from build123d import *

# Parameters (mm, degrees)
SKETCH1_W           = 60
SKETCH1_H           = 40
BOSS_EXTRUDE1_DEPTH = 6
SKETCH3_R           = 1.15
CUT_EXTRUDE2_DEPTH  = 73.360210061
SKETCH12_W          = 25
SKETCH12_H          = 54
CUT_EXTRUDE10_DEPTH = 4
CUT_EXTRUDE11_DEPTH = 2.8
FILLET1_R           = 1
SKETCH15_W          = 9
SKETCH15_H          = 4
CUT_EXTRUDE13_DEPTH = 1.8
SKETCH16_W          = 4
SKETCH16_H          = 5
BOSS_EXTRUDE2_DEPTH = 7
SKETCH17_W          = 2
SKETCH17_H          = 2
SKETCH17_W_2        = 1.8
SKETCH17_H_2        = 7
BOSS_EXTRUDE3_DEPTH = 5


with BuildPart() as part:
    # Sketch1 → Boss-Extrude1 (new body)
    with BuildSketch(Plane(origin=(0, 0, 0), x_dir=(0, 1, 0), z_dir=(0, 0, 1))):
        with Locations((30, -20)):
            Rectangle(SKETCH1_W, SKETCH1_H)
    extrude(amount=BOSS_EXTRUDE1_DEPTH)

    # Sketch3 → Cut-Extrude2 (cut, through all)
    with BuildSketch(Plane.XY.offset(6)):
        with Locations((5, 4.5)):
            Circle(SKETCH3_R)
        with Locations((35, 4.5)):
            Circle(SKETCH3_R)
        with Locations((5, 55.5)):
            Circle(SKETCH3_R)
        with Locations((35, 55.5)):
            Circle(SKETCH3_R)
    extrude(amount=-CUT_EXTRUDE2_DEPTH, mode=Mode.SUBTRACT)

    # Sketch12 → Cut-Extrude10 (cut)
    with BuildSketch(Plane.XY.offset(6)):
        with Locations((20, 29)):
            Rectangle(SKETCH12_W, SKETCH12_H)
    extrude(amount=-CUT_EXTRUDE10_DEPTH, mode=Mode.SUBTRACT)

    # Sketch13 → Cut-Extrude11 (cut)
    with BuildSketch(Plane(origin=(0, 0, 0), x_dir=(1, 0, 0), z_dir=(0, 0, -1))):
        Polygon((7.424871131, -55.5), (6.212435565, -53.4), (3.787564435, -53.4), (2.575128869, -55.5), (3.787564435, -57.6), (6.212435565, -57.6), align=None)
        Polygon((32.575128869, -55.5), (33.787564435, -57.6), (36.212435565, -57.6), (37.424871131, -55.5), (36.212435565, -53.4), (33.787564435, -53.4), align=None)
        Polygon((7.424871131, -4.5), (6.212435565, -2.4), (3.787564435, -2.4), (2.575128869, -4.5), (3.787564435, -6.6), (6.212435565, -6.6), align=None)
        Polygon((32.575128869, -4.5), (33.787564435, -6.6), (36.212435565, -6.6), (37.424871131, -4.5), (36.212435565, -2.4), (33.787564435, -2.4), align=None)
    extrude(amount=-CUT_EXTRUDE11_DEPTH, mode=Mode.SUBTRACT)

    # Fillet1
    fillet1_edges = [part.edges().sort_by_distance(p)[0] for p in [
        (0, 30, 0),
        (20, 60, 0),
        (40, 30, 0),
        (20, 0, 0),
    ]]
    fillet(fillet1_edges, radius=FILLET1_R)

    # Sketch15 → Cut-Extrude13 (cut)
    with BuildSketch(Plane.XY.offset(6)):
        with Locations((20, 58)):
            Rectangle(SKETCH15_W, SKETCH15_H)
    extrude(amount=-CUT_EXTRUDE13_DEPTH, mode=Mode.SUBTRACT)

    # Sketch16 → Boss-Extrude2 (add)
    with BuildSketch(Plane.XY.offset(2)):
        with Locations((20, 33)):
            Rectangle(SKETCH16_W, SKETCH16_H)
    extrude(amount=BOSS_EXTRUDE2_DEPTH)

    # Sketch17 → Boss-Extrude3 (add)
    with BuildSketch(Plane.XY.offset(2)):
        with Locations((20, 39.5)):
            Rectangle(SKETCH17_W, SKETCH17_H)
        with Locations((14.6, 52.5)):
            Rectangle(SKETCH17_W_2, SKETCH17_H_2)
        with Locations((25.4, 52.5)):
            Rectangle(SKETCH17_W_2, SKETCH17_H_2)
    extrude(amount=BOSS_EXTRUDE3_DEPTH)


solid = part.part
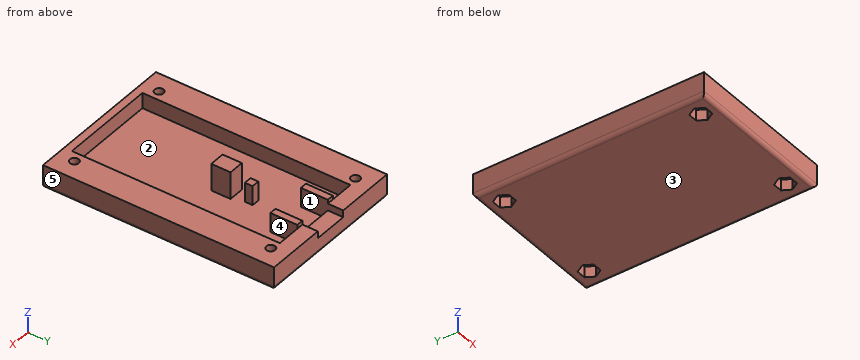
The model under review builds one solid part; all positions refer to its coordinate system, in mm. Face numbers are marked on the shaded views. A direction names the side the tool comes from. Coordinates: 2 decimals unless noted, no trailing zeros. Loops run counter-clockwise (first coordinate to the right, second up) from the corner with the lowest first, then second, coordinate; pieces in that order, holes last. Notation, with made-up numbers: (36.5, -39.5) -> (93.5, -39.5) arc R27 ccw to (93.5, -2.5) -> close; hole circle Ø5 at (26.25, -35). An arc over 180 degrees is marked (long way). Use a Markdown table: item, result. Add a question column.
1. To check wall thickness, follow line 1 (Y direction, x = 5, z = 4.2); line 2 (Y direction, x = 20.5, z = 6.5); line 3 (X direction, y = 39, z = 2.5). State the ranges of each line that lie inside material, in increasing order.
2. Add section D-D on z = 8. Write out the cut boundary in (x, y), plus the area to 3 significant figures.
3. Add section A-A on x = 35. Write out the cut boundary in (y, z), plus the area to 3 significant figures.
4. Machinability: for the marked faces 4 and 5, which of the approach directions +Z, -Z, +X, -X, +Y, -Y give a long, thin tool a straight path to every point of the face, cutting with its end or side? Answer none if there is none.
5. Draft analysis for pull direction Y (two halves, no side actions). For the marked faces 1, 2 and 3, state which applies: pulls with the +Y half, pulls with the -Y half, needs draft (parallel to the pull), parting line crosses it, or undercut.
6. Add section B-B on y = 46. Write out the cut boundary in (x, z).
7. Add section C-C on x = 9. Write out the cut boundary in (y, z).
8. Clearance check with flat-ended pins moving along their axes: pin 1 Ø2 at (x, z) = (19, 6.5) entering from -Y; pin 2 Ø3.5 at (x, y) = (5, 55.5) entering from -Z; pin 3 Ø0.8 at (x, z) = (14.5, 6.5) entering from +Y; pin 4 Ø6 at (x, y) = (5.5, 25.5) entering from +Z. State where each tip first meets the part, or that it passes through.
Returned:
| question | item | result |
|---|---|---|
| 1 | line 1 | y = 0 to 3.35, 5.65 to 54.35, 56.65 to 60 |
| 1 | line 2 | y = 30.5 to 35.5, 38.5 to 40.5 |
| 1 | line 3 | x = 0 to 7.5, 19 to 21, 32.5 to 40 |
| 2 | outline | (18, 30.5) -> (22, 30.5) -> (22, 35.5) -> (18, 35.5) -> close |
| 2 | area | 20.0 mm² |
| 3 | outline | (0, 1) arc R1 ccw to (1, 0) -> (2.4, 0) -> (2.4, 2.8) -> (3.35, 2.8) -> (3.35, 6) -> (0, 6) -> close; (5.65, 2.8) -> (6.6, 2.8) -> (6.6, 0) -> (53.4, 0) -> (53.4, 2.8) -> (54.35, 2.8) -> (54.35, 6) -> (5.65, 6) -> close; (56.65, 2.8) -> (57.6, 2.8) -> (57.6, 0) -> (59, 0) arc R1 ccw to (60, 1) -> (60, 6) -> (56.65, 6) -> close |
| 3 | area | 321 mm² |
| 4 | face 4 | +Z |
| 4 | face 5 | +Z, -Z, +X, +Y, -Y |
| 5 | face 1 | undercut |
| 5 | face 2 | undercut |
| 5 | face 3 | needs draft |
| 6 | outline | (0, 1) arc R1 ccw to (1, 0) -> (39, 0) arc R1 ccw to (40, 1) -> (40, 6) -> (32.5, 6) -> (32.5, 2) -> (7.5, 2) -> (7.5, 6) -> (0, 6) -> close |
| 7 | outline | (0, 1) arc R1 ccw to (1, 0) -> (59, 0) arc R1 ccw to (60, 1) -> (60, 6) -> (56, 6) -> (56, 2) -> (2, 2) -> (2, 6) -> (0, 6) -> close |
| 8 | pin 1 | stops at y = 0 |
| 8 | pin 2 | stops at z = 2.8 |
| 8 | pin 3 | stops at y = 56 |
| 8 | pin 4 | stops at z = 6 |
